Design review of the part shown in the three views and the two pictorial views. Dimensions are in mm from the part's minimum x, y and z. A direction names the side the tool comes from. Give positions to 0.01 mm unless a question says otherwise; leave off trailing zeros. Loops run counter-clockwise (first coordinate to the right, second up) from the corner with the lowest first, then second, coordinate; pieces in that order, holes last. Notation, with made-up numbers: (-7.5, 1.5) - (15.5, 1.5) arc R25 cw to (15.5, 26.5) - close; hole circle Ø4 at (38, 27). An arc over 180 degrees is marked (long way). Answer as a JSON object with one key per item and string values.
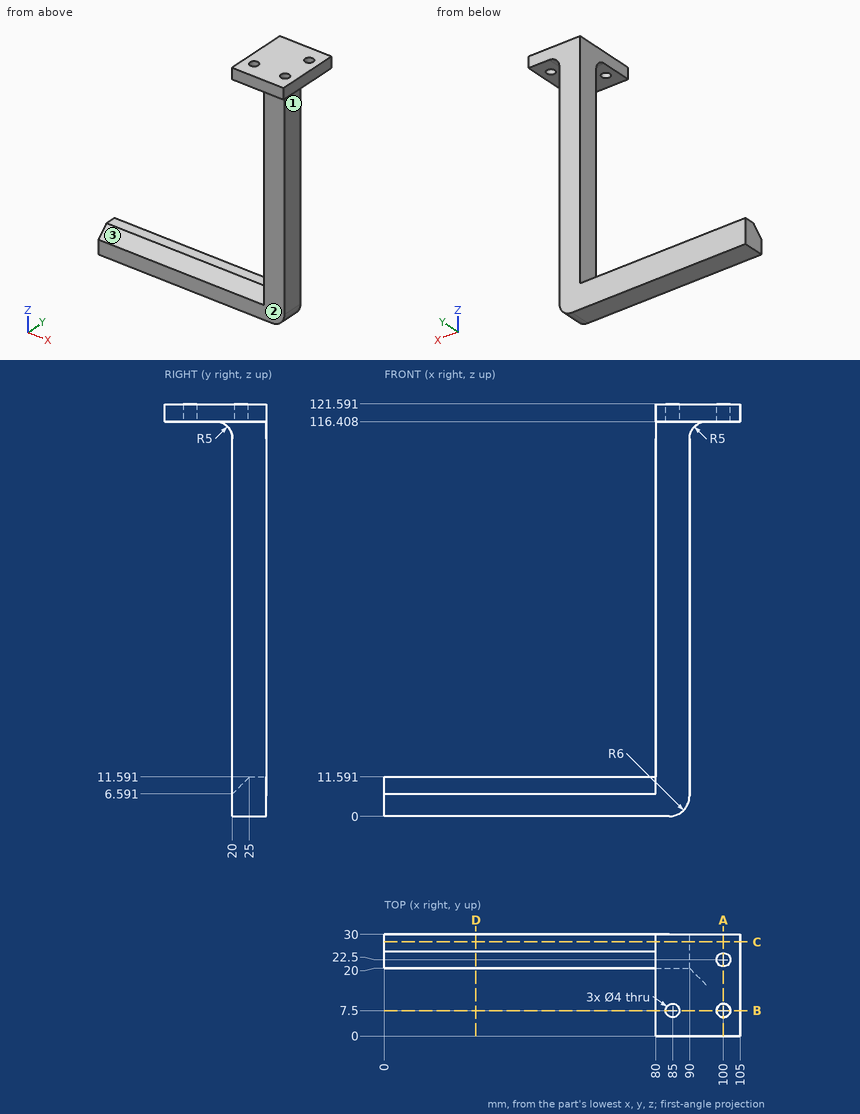
Q1. Consider section D-D, the plane x = 27. State the section outline as (y, z) points, plus the area to 3 significant figures.
Results:
{"outline": "(20, 0) - (30, 0) - (30, 11.59) - (25, 11.59) - (20, 6.59) - close", "area": "103 mm^2"}
Q2. Clearance check with flat-ended pins moving along their axes: pin 1 Ø1.5 at (x, y) = (39, 27) entering from +Z; pin 2 Ø12 at (y, z) = (25, 105.5) entering from +X; pin 3 Ø15 at (y, z) = (20, 49.5) entering from -X. State where each tip first meets the part, or that it passes through.
Results:
{"pin 1": "stops at z = 11.59", "pin 2": "stops at x = 90", "pin 3": "stops at x = 80"}
Q3. Consider section C-C, the plane y = 27.75. State the section outline as (x, z) points, plus the area to 3 significant figures.
Results:
{"outline": "(0, 0) - (84, 0) arc R6 ccw to (90, 6) - (90, 111.41) arc R5 cw to (95, 116.41) - (105, 116.41) - (105, 121.59) - (80, 121.59) - (80, 11.59) - (0, 11.59) - close", "area": "2,220 mm^2"}
Q4. For the marked faces 1, 2 and 3, list the 3-axis set-ups (+Z, -Z, +X, -X, +Y, -Y) from which the entire face can be reached by the end or side of a thin tool; tool diameter is ignored.
Results:
{"face 1": "-Z, +X, +Y, -Y", "face 2": "-Z, +X, -X, -Y", "face 3": "+Z, -X, -Y"}
Q5. Consider section A-A, the plane x = 100. State the section outline as (y, z) points, plus the area to 3 significant figures.
Results:
{"outline": "(0, 116.41) - (5.5, 116.41) - (5.5, 121.59) - (0, 121.59) - close; (9.5, 116.41) - (20.5, 116.41) - (20.5, 121.59) - (9.5, 121.59) - close; (24.5, 116.41) - (30, 116.41) - (30, 121.59) - (24.5, 121.59) - close", "area": "114 mm^2"}
Q6. Consider section B-B, the plane y = 7.5. State the section outline as (x, z) points.
Results:
{"outline": "(80, 116.41) - (83, 116.41) - (83, 121.59) - (80, 121.59) - close; (87, 116.41) - (98, 116.41) - (98, 121.59) - (87, 121.59) - close; (102, 116.41) - (105, 116.41) - (105, 121.59) - (102, 121.59) - close"}
Q7. To check wall thickness, follow probe 1 along Y at (x, z) = (100, 119.75); probe 2 along Y at (x, z) = (85, 118); probe 3 along Z at (x, y) = (86, 5.25). State the ranges of each line that lie inside material, in increasing order. Write a range as [from, to].
Results:
{"probe 1": "y = [0, 5.5], [9.5, 20.5], [24.5, 30]", "probe 2": "y = [0, 5.5], [9.5, 30]", "probe 3": "z = [116.41, 121.59]"}
